```python
from build123d import *

# Parameters (mm, degrees)
SKETCH1_R           = 0.75
SKETCH1_R_2         = 1.5
BOSS_EXTRUDE1_DEPTH = 2.5
SKETCH2_R           = 4.25
SKETCH2_R_2         = 3
BOSS_EXTRUDE2_DEPTH = 4
SKETCH3_R           = 4.5
CUT_EXTRUDE1_DEPTH  = 0.8
SKETCH4_R           = 3.7
SKETCH4_R_2         = 3.5
BOSS_EXTRUDE3_DEPTH = 1
FILLET2_R           = 0.5
FILLET3_R           = 0.2


with BuildPart() as part:
    # Sketch1 → Boss-Extrude1 (new body)
    with BuildSketch(Plane.XY):
        with BuildLine():
            Line((1.934972164, 16.505848487), (5.247058111, 3.836454246))
            ThreePointArc((5.247058111, 3.836454246), (6.499999994, -0.000272762), (5.246736111, -3.836894601))
            Line((5.246736111, -3.836894601), (1.919269062, -16.5625))
            ThreePointArc((1.919269062, -16.5625), (0, -17.999999995), (-1.919269062, -16.562499999))
            Line((-1.919269062, -16.562499999), (-5.246736111, -3.836894601))
            ThreePointArc((-5.246736111, -3.836894601), (-6.499999994, -0.000272762), (-5.247058111, 3.836454246))
            Line((-5.247058111, 3.836454246), (-1.934972164, 16.505848487))
            ThreePointArc((-1.934972164, 16.505848487), (0, 17.999999979), (1.934972164, 16.505848487))
        make_face()
        with Locations((0, 7)):
            Circle(SKETCH1_R, mode=Mode.SUBTRACT)
        with Locations((0, 10)):
            Circle(SKETCH1_R, mode=Mode.SUBTRACT)
        with Locations((0, 13)):
            Circle(SKETCH1_R, mode=Mode.SUBTRACT)
        with Locations((0, 16)):
            Circle(SKETCH1_R, mode=Mode.SUBTRACT)
        Circle(SKETCH1_R_2, mode=Mode.SUBTRACT)
        with Locations((0, -16)):
            Circle(SKETCH1_R, mode=Mode.SUBTRACT)
        with Locations((0, -13)):
            Circle(SKETCH1_R, mode=Mode.SUBTRACT)
        with Locations((0, -10)):
            Circle(SKETCH1_R, mode=Mode.SUBTRACT)
        with Locations((0, -7)):
            Circle(SKETCH1_R, mode=Mode.SUBTRACT)
    extrude(amount=BOSS_EXTRUDE1_DEPTH)

    # Sketch2 → Boss-Extrude2 (add)
    with BuildSketch(Plane.XY.offset(2.5)):
        Circle(SKETCH2_R)
        Circle(SKETCH2_R_2, mode=Mode.SUBTRACT)
    extrude(amount=BOSS_EXTRUDE2_DEPTH)

    # Sketch3 → Cut-Extrude1 (cut)
    with BuildSketch(Plane(origin=(0, 0, 0), x_dir=(-1, 0, 0), z_dir=(0, 0, -1))):
        Circle(SKETCH3_R)
    extrude(amount=-CUT_EXTRUDE1_DEPTH, mode=Mode.SUBTRACT)

    # Sketch4 → Boss-Extrude3 (add)
    with BuildSketch(Plane(origin=(0, 0, 0.8), x_dir=(-1, 0, 0), z_dir=(0, 0, -1))):
        Circle(SKETCH4_R)
        Circle(SKETCH4_R_2, mode=Mode.SUBTRACT)
    extrude(amount=BOSS_EXTRUDE3_DEPTH)

    # Fillet2
    fillet2_edges = [part.edges().sort_by_distance(p)[0] for p in [
        (-4.25, 0, 6.5),
    ]]
    fillet(fillet2_edges, radius=FILLET2_R)

    # Fillet3
    fillet3_edges = [part.edges().sort_by_distance(p)[0] for p in [
        (3.583002587, -10.1996973, 2.5),
        (0, -17.999999995, 2.5),
        (-3.583002587, -10.1996973, 2.5),
        (-3.591015137, 10.171151366, 2.5),
        (0, 17.999999979, 2.5),
        (-3.591015137, 10.171151366, 0),
        (0, 17.999999979, 0),
        (3.591015137, 10.171151366, 2.5),
        (3.591015137, 10.171151366, 0),
        (6.499999994, -0.000272762, 2.5),
        (6.499999994, -0.000272762, 0),
        (5.247058111, 3.836454246, 1.25),
        (-6.499999994, -0.000272762, 2.5),
    ]]
    fillet(fillet3_edges, radius=FILLET3_R)


solid = part.part
```
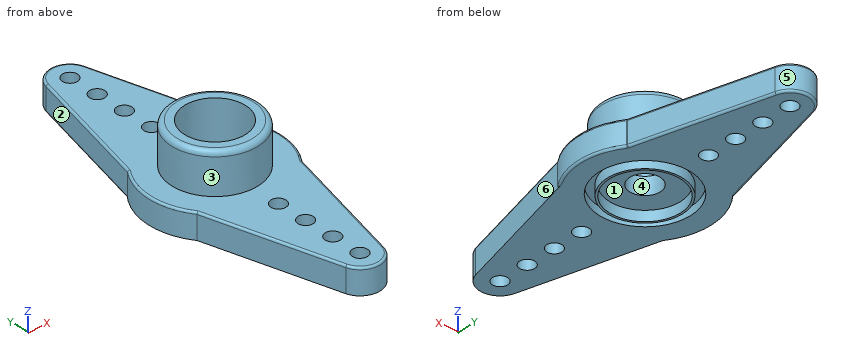
Can you work these out from the model? Positions are in its coordinate system, mm. Face numbers are marked on the shaded views. A direction names the side the tool comes from. Round coordinates to 2 decimals unless told otherwise and drop trailing zeros. Loops run counter-clockwise (first coordinate to the right, second up) from the corner with the lowest first, then second, coordinate; pieces in that order, holes last.
Item 1: Suppose I cut it at A-A, the plane z = 1.5. State how many separate pieces and enclosed holes the cut face has, then the cut area to 3 significant figures.
Item 2: Suppose I cut it at B-B, the plane z = 5. Write out the boundary of the cut face in (x, y).
Item 3: Which directions (+Z, -Z, +X, -X, +Y, -Y) give clear straight access to the entire face, cutting with the end or side of a thin tool? Please do the marked faces 1, 2 and 3.
Item 4: Please list where these lines run through material, in increasing order: L1, parallel to Y at x = -0.5, z = 2.75; L2, parallel to Z at x = -1, y = -6; L3, parallel to X at y = 16.5, z = 1.25.
Item 5: If we mould it in two halves opening along X, with no side actions, what happens to the marked faces 4, 5 and 6? For each: +X half, -X half, draft (parallel to the pull), parting line (faces both ways), or undercut.
Item 6: Will these pins go through, and if not, where does the flat tip stop? pin 1 Ø2 at (x, y) = (0, -13) entering from +Z; pin 2 Ø3.5 at (x, y) = (1, 0) entering from -Z; pin 3 Ø2.5 at (x, y) = (0, 13) entering from -Z; pin 4 Ø5 at (x, y) = (0, 1.5) entering from +Z.
Reported:
1. separate pieces: 1
1. enclosed holes: 9
1. area: 263 mm2
2. outline: circle Ø8.5 at (0, 0); hole circle Ø6 at (0, 0)
3. face 1: -Z
3. face 2: +Z, -Z, -X, +Y
3. face 3: +Z
4. L1: y = -4.22 to -2.96, 2.96 to 4.22
4. L2: z = 0 to 2.5
4. L3: x = -1.94 to -0.56, 0.56 to 1.94
5. face 4: undercut
5. face 5: parting line
5. face 6: +X half
6. pin 1: stops at z = 2.5
6. pin 2: stops at z = 0.8
6. pin 3: stops at z = 0
6. pin 4: stops at z = 6.5
